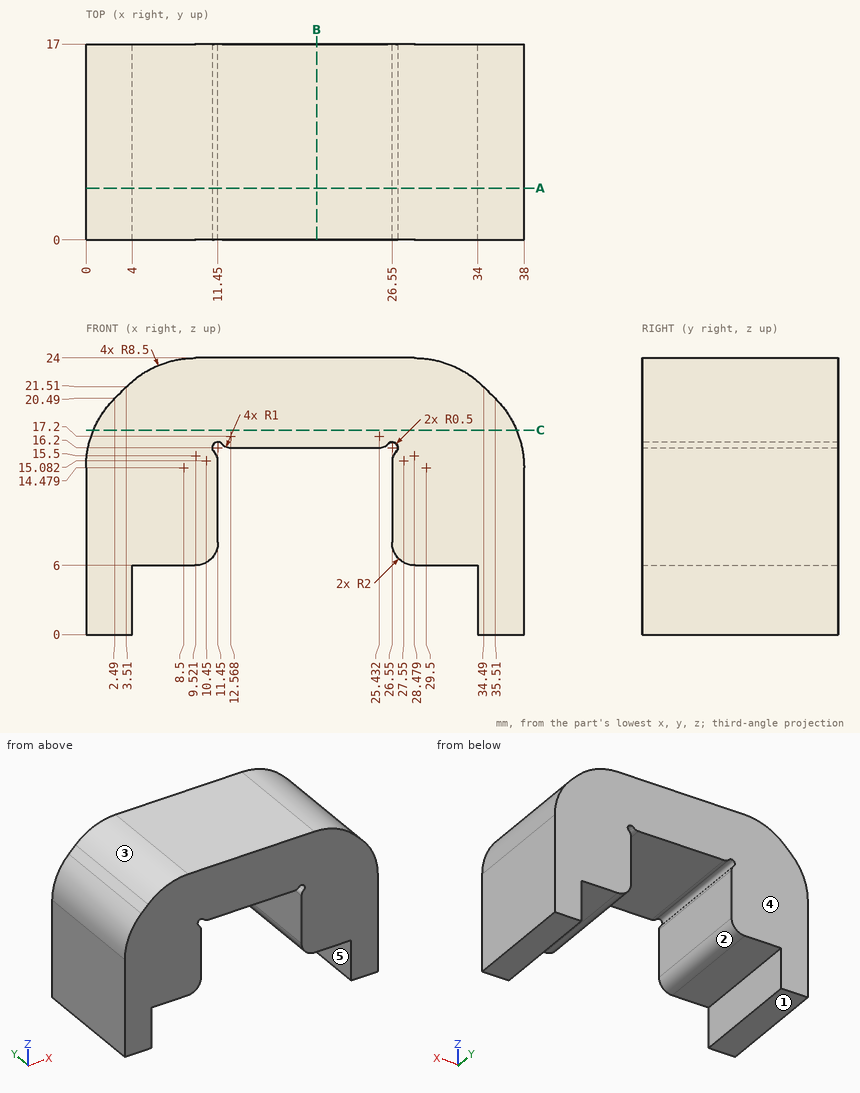
For this review, use the dimensioned drawing (mm, ordinates from the lowest corner) and the shaded views. A direction names the side the tool comes from. Coordinates: 2 decimals unless noted, no trailing zeros. Order: outer loops, then holes, each group sorted by start corner. A loop starts at its lowest first (then second) coordinate and runs counter-clockwise, first axis right, second up. Notation, with made-up numbers: (24.5, 5.5) -> (32.5, 5.5) arc R13 cw to (32.5, 10.5) -> close; hole circle Ø4 at (-23.5, -32). An arc over 180 degrees is marked (long way). One line per item, written item: value. Start each with the question number.
Q1. For probe 1 along X at (y, z) = (8.25, 11); probe 2 along Z at (x, y) = (24, 10.5); probe 3 along X at (y, z) = (12.5, 7.25) (1 decimal), list the stretches that pass through material, from the lowest coordinate up.
Q2. Insertion check: pin 1 Ø4.5 at (x, y) = (7.5, 5) entering from -Z. The pin has a flat end and moves straight along its axis. Give the tip position at first contact, or say it passes through.
Q3. Take a section at A-A, the plane y = 4.5. State the section outline as (x, z) points.
Q4. Tool access review of the marked faces 4 and 5: name each direction out of +Z, -Z, +X, -X, +Y, -Y from which nothing blocks a thin tool from reaching the whole face with its end or side.
Q5. Take a section at B-B, the plane x = 20. State the section outline as (y, z) points.
Q6. Take a section at C-C, the plane z = 17.75. State the section outline as (x, y) points (1 decimal), then the cut area to 3 significant figures.
Q7. Mouldability with a two-part tool opening along X and no side actions: class the marked faces 1, 2 and 3 as pulls with the +X half, pulls with the -X half, needs draft (parallel to the pull), parting line crosses it, or undercut.
Values follow:
1. probe 1: x = 0 to 11.45, 26.55 to 38
1. probe 2: z = 16.2 to 24
1. probe 3: x = 0 to 11.3, 26.7 to 38
2. pin 1: stops at z = 6
3. outline: (0, 0) -> (4, 0) -> (4, 6) -> (9.45, 6) arc R2 ccw to (11.45, 8) -> (11.45, 15.08) arc R1 ccw to (11.12, 15.83) arc R0.5 cw (long way) to (11.82, 16.53) arc R1 ccw to (12.57, 16.2) -> (25.43, 16.2) arc R1 ccw to (26.18, 16.53) arc R0.5 cw (long way) to (26.88, 15.83) arc R1 ccw to (26.55, 15.08) -> (26.55, 8) arc R2 ccw to (28.55, 6) -> (34, 6) -> (34, 0) -> (38, 0) -> (38, 14.48) arc R8.5 ccw to (35.51, 20.49) -> (34.49, 21.51) arc R8.5 ccw to (28.48, 24) -> (9.52, 24) arc R8.5 ccw to (3.51, 21.51) -> (2.49, 20.49) arc R8.5 ccw to (0, 14.48) -> close
4. face 4: +Z, -Z, +X, -X, +Y
4. face 5: -Z, +Y, -Y
5. outline: (0, 16.2) -> (17, 16.2) -> (17, 24) -> (0, 24) -> close
6. outline: (0.7, 0) -> (37.3, 0) -> (37.3, 17) -> (0.7, 17) -> close
6. area: 624 mm2
7. face 1: needs draft
7. face 2: undercut
7. face 3: pulls with the -X half
